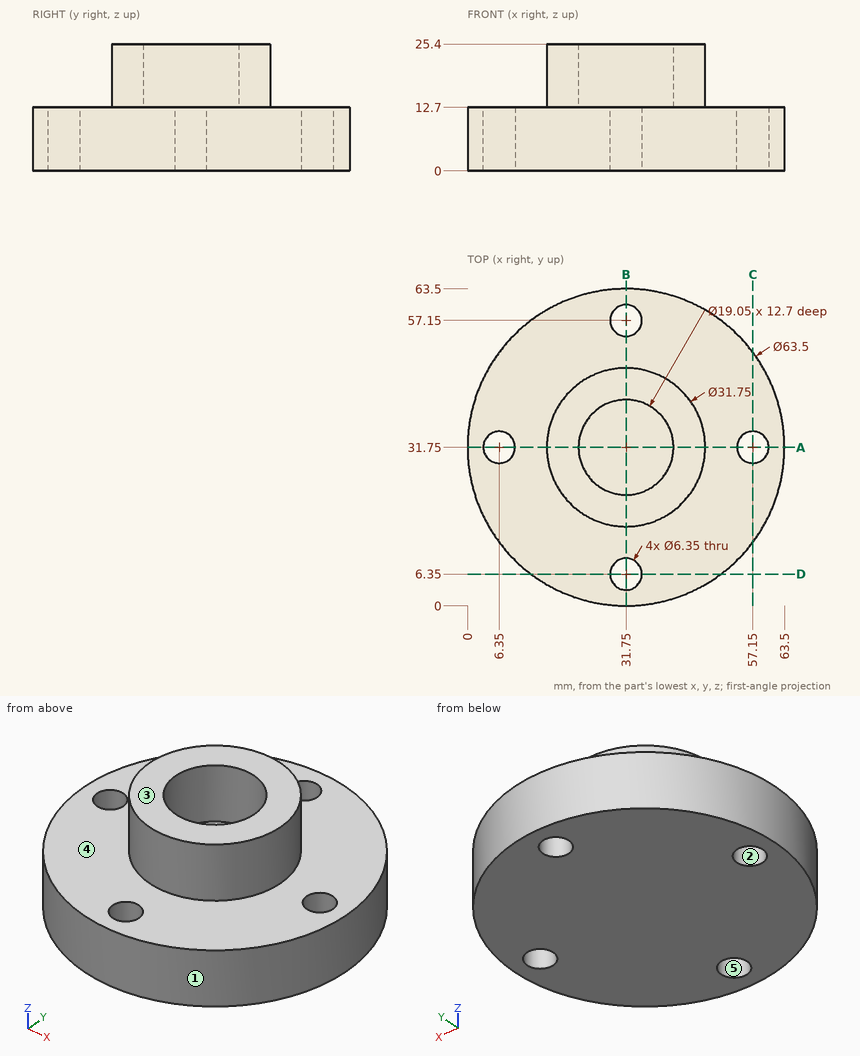
Print and shaded views of the part. All mm, measured from the part's lowest x, y and z. A direction names the side the tool comes from. Give positions to 0.01 mm unless a question says otherwise; leave off trailing zeros. Order: outer loops, then holes, each group sorted by start corner. A loop starts at its lowest first (then second) coordinate and runs counter-clockwise, first axis right, second up. Notation, with made-up numbers: (30.25, -37) - (79.25, -37) arc R23 cw to (79.25, -1) - close; hole circle Ø7 at (26, 28). An arc over 180 degrees is marked (long way). One line per item, written item: value.
Item 1: Wall check: line 1 (Y direction, x = 31.75, z = 7.75) (3 decimals); line 2 (Y direction, x = 31.75, z = 21.5) (3 decimals); line 3 (Z direction, x = 24.5, y = 9). Give the ranges that are in metal, low to high.
Response values:
line 1: 0 to 3.175, 9.525 to 53.975, 60.325 to 63.5
line 2: 15.875 to 22.225, 41.275 to 47.625
line 3: 0 to 12.7
Item 2: Two-plate mould, pull along Y, no slides. Class the marked faces 1, 2 and 3: released by +Y, released by -Y, zero draft, split by the parting line, or undercut.
Response values:
face 1: split by the parting line
face 2: undercut
face 3: zero draft
Item 3: Slice it at C-C (x = 57.15). List the corners of the cut face in (y, z) (3 decimals), then the cut area to 3 significant figures.
Response values:
outline: (12.7, 0) - (28.575, 0) - (28.575, 12.7) - (12.7, 12.7) - close; (34.925, 0) - (50.8, 0) - (50.8, 12.7) - (34.925, 12.7) - close
area: 403 mm2
Item 4: Slice it at A-A (y = 31.75). List the corners of the cut face in (x, z) (3 decimals).
Response values:
outline: (0, 0) - (3.175, 0) - (3.175, 12.7) - (0, 12.7) - close; (9.525, 0) - (53.975, 0) - (53.975, 12.7) - (47.625, 12.7) - (47.625, 25.4) - (41.275, 25.4) - (41.275, 12.7) - (22.225, 12.7) - (22.225, 25.4) - (15.875, 25.4) - (15.875, 12.7) - (9.525, 12.7) - close; (60.325, 0) - (63.5, 0) - (63.5, 12.7) - (60.325, 12.7) - close
Item 5: Pin check, flat tips, straight feed: pin 1 Ø5 at (x, z) = (53, 12) entering from +Y; pin 2 Ø7.5 at (x, y) = (57.15, 31.75) entering from +Z; pin 3 Ø3 at (x, z) = (13.5, 9.5) entering from +Y. Stop position of each tip, or through.
Response values:
pin 1: y = 57.37
pin 2: z = 12.7
pin 3: y = 58.72
Item 6: Tool access for the marked faces 4 and 5: list every direction of +Z, -Z, +X, -X, +Y, -Y with a clear straight run to the whole face (end or side of a thin tool).
Response values:
face 4: +Z
face 5: +Z, -Z
